Geometry check sheet. Reference: the model listing, model coordinates, mm. Round coordinates to 2 decimals unless told otherwise and drop trailing zeros. Order: outer loops, then holes, each group sorted by start corner. A loop starts at its lowest first (then second) coordinate and runs counter-clockwise, first axis right, second up.
(1) Cross-section at B-B on x = 22. Enter the section's corners in (y, z).
(2) Gauge pin test, flat end, axial feed: P1, Ø1.2, axis at x = 22, y = -8, coming from the +Z side. Record the tip position at first contact, or that the pin passes through.
(3) Cross-section at A-A on y = -8. Enter the section's corners in (x, z).
(4) Draft check along X on faces 1 (the face through (21, -8, 3)), 2 (the face through (0, 0, 0)), 3 (the face through (24.43, 10.4, 2.79)). Enter one of: pulls with the +X half, pulls with the -X half, needs draft (parallel to the pull), parting line crosses it, or undercut.
(5) Thickness scan on L1, parallel to Y at x = -22, z = 2.2; L2, parallel to X at y = 8, z = 3.85; L3, parallel to X at y = -8.75, z = 1.55. Record the ranges inside material, lowest first.
Solid Edge part; units mm, degrees
sketch "Sketch1" plane through (0, 0, 0) normal (0, 0, 1) x (1, 0, 0)
  line L0 (25, 11) -> (-25, 11)
  line L1 (-25, 11) -> (-25, -11)
  line L2 (-25, -11) -> (25, -11)
  line L3 (25, -11) -> (25, 11)
  dimension "D1" = 25
  dimension "D2" = 25
extrude "Protrusion1" add sketch "Sketch1" along normal blind 5.5
hole "Hole_1" at (-22, 8, 5.5) direction (0, 0, -1) diameter 2 end through all
hole "Hole1" at (-22, -8, 5.5) direction (0, 0, -1) diameter 2 end through all
hole "Hole2" at (22, -8, 5.5) direction (0, 0, -1) diameter 2 end through all
hole "Hole3" at (22, 8, 5.5) direction (0, 0, -1) diameter 2 end through all
fillet "Round_1" radius 2 4 edges at (-25, 11, 2.75) (-25, -11, 2.75) (25, -11, 2.75) (25, 11, 2.75)
properties material "木材, アッシュ"
Found:
1. outline: (-11, 0) - (-9, 0) - (-9, 5.5) - (-11, 5.5) - close; (-7, 0) - (7, 0) - (7, 5.5) - (-7, 5.5) - close; (9, 0) - (11, 0) - (11, 5.5) - (9, 5.5) - close
2. P1: passes through
3. outline: (-25, 0) - (-23, 0) - (-23, 5.5) - (-25, 5.5) - close; (-21, 0) - (21, 0) - (21, 5.5) - (-21, 5.5) - close; (23, 0) - (25, 0) - (25, 5.5) - (23, 5.5) - close
4. face 1: undercut
4. face 2: needs draft
4. face 3: pulls with the +X half
5. L1: y = -11 to -9, -7 to 7, 9 to 11
5. L2: x = -25 to -23, -21 to 21, 23 to 25
5. L3: x = -25 to -22.66, -21.34 to 21.34, 22.66 to 25
